Work out the finished part from the listing and answer in its coordinate system (mm). A direction names the side the tool comes from. Give positions to 0.01 mm unless a question says otherwise; leave off trailing zeros. Loops run counter-clockwise (first coordinate to the right, second up) from the corner with the lowest first, then second, coordinate; pieces in that order, holes last. Notation, with made-up numbers: M 44.25,-3.75 L 52.25,-3.75 A21 cw 52.25,1.25 Z; hole C 18,80.5 d9. An arc over 180 degrees is marked long. Answer as a JSON object with one key per item and string values. Group by question number.
```python
from build123d import *

# Parameters (mm, degrees)
EXTRUDE002_DEPTH = 2.5
BOX001_W         = 53
BOX001_H         = 46
BOX001_DEPTH     = 5
BOX002_W         = 5
BOX002_H         = 30
BOX002_DEPTH     = 12
BOX003_W         = 5
BOX003_H         = 30
BOX003_DEPTH     = 12
BOX_W            = 53
BOX_H            = 5
BOX_DEPTH        = 60
SKETCH028_R      = 1.75
SKETCH028_R_2    = 13.25
POCKET001_DEPTH  = 5
CHAMFER_SIZE     = 8
CHAMFER001_SIZE  = 4
SKETCH029_W      = 16.5
SKETCH029_H      = 46
POCKET002_DEPTH  = 1.5
CHAMFER002_SIZE  = 5
CHAMFER003_SIZE  = 5
POCKET003_DEPTH  = 5
POCKET004_DEPTH  = 3
SKETCH032_W      = 37
SKETCH032_H      = 26.5
POCKET005_DEPTH  = 5
SKETCH033_W      = 3
SKETCH033_H      = 47.5
PAD003_DEPTH     = 1
SKETCH034_W      = 8
SKETCH034_H      = 8.75
SKETCH034_R      = 1.75
SKETCH034_H_2    = 10.75
PAD004_DEPTH     = 4
SKETCH035_W      = 16.5
SKETCH035_H      = 4
POCKET006_DEPTH  = 2
CHAMFER004_SIZE  = 4.99
CHAMFER005_SIZE  = 3.99
CHAMFER006_SIZE  = 2


with BuildPart() as extrude002:
    # Facebinder → Extrude002 (new body)
    with BuildSketch(Plane(origin=(40.336531, -57.03076, 116), x_dir=(0, 1, 0), z_dir=(0, 0, 1))):
        Polygon((-18.96924, 7.336531), (-23.96924, 2.336531), (-23.96924, -10.913469), (-15.21924, -10.913469), (-15.21924, -0.663469), (11.28076, -0.663469), (11.28076, -10.913469), (22.03076, -10.913469), (22.03076, 7.336531), align=None)
        Polygon((-23.96924, -40.663469), (-18.96924, -45.663469), (22.03076, -45.663469), (22.03076, -27.413469), (11.28076, -27.413469), (11.28076, -37.663469), (-15.21924, -37.663469), (-15.21924, -27.413469), (-23.96924, -27.413469), align=None)
    extrude(amount=EXTRUDE002_DEPTH)


with BuildPart() as box001:
    # Box001 → Box001 (new body)
    with BuildSketch(Plane(origin=(33, -76, 111), x_dir=(1, 0, 0), z_dir=(0, 0, 1))):
        with Locations((26.5, 23)):
            Rectangle(BOX001_W, BOX001_H)
    extrude(amount=BOX001_DEPTH)


with BuildPart() as box002:
    # Box002 → Box002 (new body)
    with BuildSketch(Plane(origin=(81, -56, 102), x_dir=(1, 0, 0), z_dir=(0, 0, 1))):
        with Locations((2.5, 15)):
            Rectangle(BOX002_W, BOX002_H)
    extrude(amount=BOX002_DEPTH)


with BuildPart() as box003:
    # Box003 → Box003 (new body)
    with BuildSketch(Plane(origin=(33, -56, 102), x_dir=(1, 0, 0), z_dir=(0, 0, 1))):
        with Locations((2.5, 15)):
            Rectangle(BOX003_W, BOX003_H)
    extrude(amount=BOX003_DEPTH)


with BuildPart() as chamfer006:
    # Box → Box (new body)
    with BuildSketch(Plane(origin=(33, -30, 102), x_dir=(1, 0, 0), z_dir=(0, 0, 1))):
        with Locations((26.5, 2.5)):
            Rectangle(BOX_W, BOX_H)
    extrude(amount=BOX_DEPTH)

    # Fusion001: union Box001, Box002, Box003
    add(box001.part)
    add(box002.part)
    add(box003.part)


with BuildPart() as chamfer006_1:
    # Fusion001 placement: moved
    add(chamfer006.part.moved(Location((0, -5, 0))))

    # Sketch028 → Pocket001 (cut)
    with BuildSketch(Plane(origin=(0, -5, 116), x_dir=(1, 0, 0), z_dir=(0, 0, 1))):
        with Locations((59.5, -70)):
            Circle(SKETCH028_R)
        with Locations((59.5, -38)):
            Circle(SKETCH028_R)
        with Locations((59.5, -54)):
            Circle(SKETCH028_R_2)
    extrude(amount=-POCKET001_DEPTH, mode=Mode.SUBTRACT)

    # Chamfer
    chamfer_edges = [chamfer006_1.edges().sort_by_distance(p)[0] for p in [
        (83.5, -61, 102),
        (35.5, -61, 102),
    ]]
    chamfer(chamfer_edges, length=CHAMFER_SIZE)

    # Chamfer001
    chamfer001_edges = [chamfer006_1.edges().sort_by_distance(p)[0] for p in [
        (86, -41.5, 102),
        (33, -41.5, 102),
    ]]
    chamfer(chamfer001_edges, length=CHAMFER001_SIZE)

    # Sketch029 → Pocket002 (cut)
    with BuildSketch(Plane(origin=(0, -5, 116), x_dir=(1, 0, 0), z_dir=(0, 0, 1))):
        with Locations((59.5, -53)):
            Rectangle(SKETCH029_W, SKETCH029_H)
    extrude(amount=-POCKET002_DEPTH, mode=Mode.SUBTRACT)

    # Chamfer002
    chamfer002_edges = [chamfer006_1.edges().sort_by_distance(p)[0] for p in [
        (86, -81, 113.5),
        (33, -81, 113.5),
    ]]
    chamfer(chamfer002_edges, length=CHAMFER002_SIZE)

    # Chamfer003
    chamfer003_edges = [chamfer006_1.edges().sort_by_distance(p)[0] for p in [
        (86, -32.5, 162),
        (33, -32.5, 162),
    ]]
    chamfer(chamfer003_edges, length=CHAMFER003_SIZE)

    # Sketch030 → Pocket003 (cut)
    with BuildSketch(Plane.XZ.offset(35)):
        with BuildLine():
            Line((49.2, 151), (49.2, 127))
            ThreePointArc((45.8, 127), (47.5, 125.3), (49.2, 127))
            Line((45.8, 127), (45.8, 151.000018))
            ThreePointArc((49.2, 151), (47.500009, 152.7), (45.8, 151.000018))
        make_face()
        with BuildLine():
            Line((69.8, 151), (69.8, 127))
            ThreePointArc((69.8, 127), (71.5, 125.3), (73.2, 127))
            Line((73.2, 127), (73.2, 151))
            ThreePointArc((73.2, 151), (71.5, 152.7), (69.8, 151))
        make_face()
    extrude(amount=-POCKET003_DEPTH, mode=Mode.SUBTRACT)

    # Sketch031 → Pocket004 (cut)
    with BuildSketch(Plane.XZ.offset(35)):
        with BuildLine():
            ThreePointArc((50.9, 151), (47.5, 154.4), (44.1, 151))
            Line((44.1, 151), (44.1, 127))
            ThreePointArc((44.1, 127), (47.5, 123.6), (50.9, 127))
            Line((50.9, 151), (50.9, 127))
        make_face()
        with BuildLine():
            ThreePointArc((74.9, 151), (71.5, 154.4), (68.1, 151))
            Line((68.1, 151), (68.1, 127))
            ThreePointArc((68.1, 127), (71.5, 123.6), (74.9, 127))
            Line((74.9, 151), (74.9, 127))
        make_face()
    extrude(amount=-POCKET004_DEPTH, mode=Mode.SUBTRACT)

    # Sketch032 → Pocket005 (cut)
    with BuildSketch(Plane(origin=(0, -5, 116), x_dir=(1, 0, 0), z_dir=(0, 0, 1))):
        with Locations((59.5, -54)):
            Rectangle(SKETCH032_W, SKETCH032_H)
    extrude(amount=-POCKET005_DEPTH, mode=Mode.SUBTRACT)

    # Fusion002: union Extrude002
    add(extrude002.part)

    # Sketch033 → Pad003 (new body)
    with BuildSketch(Plane.XZ.offset(35)):
        Polygon((33, 118.5), (36, 118.5), (36, 156.631975), (36, 160), (33, 157), align=None)
        Polygon((86, 118.5), (83, 118.5), (83, 156.631975), (83, 160), (86, 157), align=None)
        with Locations((59.5, 138.25)):
            Rectangle(SKETCH033_W, SKETCH033_H)
    extrude(amount=PAD003_DEPTH)

    # Sketch034 → Pad004 (new body)
    with BuildSketch(Plane(origin=(0, 0, 111), x_dir=(1, 0, 0), z_dir=(0, 0, -1))):
        with Locations((59.5, 76.625)):
            Rectangle(SKETCH034_W, SKETCH034_H)
        with Locations((59.5, 75)):
            Circle(SKETCH034_R, mode=Mode.SUBTRACT)
        with Locations((59.5, 40.375)):
            Rectangle(SKETCH034_W, SKETCH034_H_2)
        with Locations((59.5, 43)):
            Circle(SKETCH034_R, mode=Mode.SUBTRACT)
    extrude(amount=PAD004_DEPTH)

    # Sketch035 → Pocket006 (cut)
    with BuildSketch(Plane.XZ.offset(36)):
        with Locations((59.5, 116.5)):
            Rectangle(SKETCH035_W, SKETCH035_H)
    extrude(amount=-POCKET006_DEPTH, mode=Mode.SUBTRACT)

    # Chamfer004
    chamfer004_edges = [chamfer006_1.edges().sort_by_distance(p)[0] for p in [
        (59.5, -35, 107),
    ]]
    chamfer(chamfer004_edges, length=CHAMFER004_SIZE)

    # Chamfer005
    chamfer005_edges = [chamfer006_1.edges().sort_by_distance(p)[0] for p in [
        (63.5, -76.625, 111),
        (63.5, -40.375, 111),
        (55.5, -40.375, 111),
        (55.5, -76.625, 111),
    ]]
    chamfer(chamfer005_edges, length=CHAMFER005_SIZE)

    # Chamfer006
    chamfer006_edges = [chamfer006_1.edges().sort_by_distance(p)[0] for p in [
        (59.5, -81, 107),
    ]]
    chamfer(chamfer006_edges, length=CHAMFER006_SIZE)


solid = chamfer006_1.part
```
Item 1: For a pull along Z with two mould halves and no side action, classify faces 6 (the flat face through (35, -43, 104)), 7 (the flat face through (74, -32, 139)), 8 (the flat face through (38, -45, 106)) as pulls with the +Z half, pulls with the -Z half, needs draft (parallel to the pull), parting line crosses it, or undercut.
Item 2: Find the intervals of material crossed by probe 1 along Y at (x, z) = (59.5, 110.75); probe 2 along X at (y, z) = (-48.5, 110.5); probe 3 along X at (y, z) = (-75, 111.5), in increasing order. Write a range as [from, to].
Item 3: A tool of negligible diameter and unlimited length cuts with its end or side. For faces 1 (the flat face through (34, -36, 140)), 2 (the flat face through (74.9, -34, 139)), 3 (the cylindrical face through (47.5, -31, 152.7)), 4 (the flat face through (63.5, -37, 105)), 5 (the flat face through (67.75, -77, 116)), from which of +Z, -Z, +X, -X, +Y, -Y can it reach the whole face along a straight path? Write none if from no direction.
Item 4: A cutting plane is placed at C-C (x = 59.5). Give the number of separate pieces and of enclosed holes in the cut face, and give its area (3 significant figures).
Item 5: Given pin 1 Ø2.5 at (y, z) = (-38, 103.5) entering from -X; pin 2 Ø15 at (x, y) = (43.5, -66.5) entering from -Z; pin 3 Ø7.5 at (x, z) = (70, 133) entering from -Y, each flat-ended and moving along its own axis, determine where each tip first touches the part or whether it passes through.
Item 6: A cutting plane is placed at A-A (x = 71.5). Determine the outline of the cut face in (y, z), and give its area (3 significant figures).
The answers:
{
 "1": {"face 6": "pulls with the -Z half", "face 7": "undercut", "face 8": "needs draft"},
 "2": {"probe 1": "y = [-81, -76.75], [-73.25, -72.25], [-45.75, -44.75], [-41.25, -30]", "probe 2": "x = [33, 38], [81, 86]", "probe 3": "x = [33, 57.75], [61.25, 86]"},
 "3": {"face 1": "+Z, +X, -X, -Y", "face 2": "-Y", "face 3": "+Y, -Y", "face 4": "-Z, -Y", "face 5": "+Z, -Y"},
 "4": {"separate pieces": "4", "enclosed holes": "0", "area": "444 mm^2"},
 "5": {"pin 1": "stops at x = 34.25", "pin 2": "stops at z = 111", "pin 3": "stops at y = -35"},
 "6": {"outline": "M -81,111 L -72.25,111 L -72.25,118.5 L -81,118.5 Z; M -45.75,111 L -35,111 L -35,102 L -30,102 L -30,125.3 L -32,125.3 L -32,123.6 L -35,123.6 L -35,118.5 L -45.75,118.5 Z; M -35,154.4 L -32,154.4 L -32,152.7 L -30,152.7 L -30,162 L -35,162 Z", "area": "299 mm^2"}
}
